Here's the drawing with two shaded views (mm, measured from the low corner). I have some questions. Coordinates: 2 decimals unless noted, no trailing zeros. Loops run counter-clockwise (first coordinate to the right, second up) from the corner with the lowest first, then second, coordinate; pieces in that order, holes last. Notation, with made-up numbers: (-0.75, 62) -> (56.25, 62) arc R19 cw to (56.25, 88) -> close; hole circle Ø11 at (-7.5, 21). An arc over 180 degrees is marked (long way). Answer as a JSON object with one key per item and string values. Group by question number.
Q1. I want a section at A-A on x = 50.8. Count the separate pieces of the cut face and the enclosed holes in it, then the cut area to 3 significant figures.
Q2. Thinking about a two-plate mould opening in Z: for the marked faces 1, 2 and 3, which applies, released by +Z, released by -Z, zero draft, split by the parting line, or undercut?
Q3. I want a section at D-D on y = 16.75. Write out the boundary of the cut face in (x, z) (3 decimals).
Q4. I need wall thicknesses on line 1 (Z direction, x = 50.8, y = 16); line 2 (Y direction, x = 50, z = 88.9) (3 decimals); line 3 (Y direction, x = 7.5, z = 50.5). Which ranges of each line are inside material? Lowest first, please.
Q5. I want a section at C-C on x = 38.5. Write out the boundary of the cut face in (y, z).
Q6. I want a section at B-B on z = 50.8. Write out the boundary of the cut face in (x, y) (3 decimals), then the cut area to 3 significant figures.
Q7. I'm going to push flat-ended pins straight in: pin 1 (4 mm diameter, centred on y = 4.5, z = 91, fed in from +X); pin 2 (10 mm diameter, centred on x = 12.7, z = 50.8, fed in from -Y); pin 3 (1.5 mm diameter, centred on y = 11, z = 47, fed in from -X); pin 4 (6.5 mm diameter, centred on y = 3.5, z = 91, fed in from -X). Where does each tip first touch, or does it pass through?
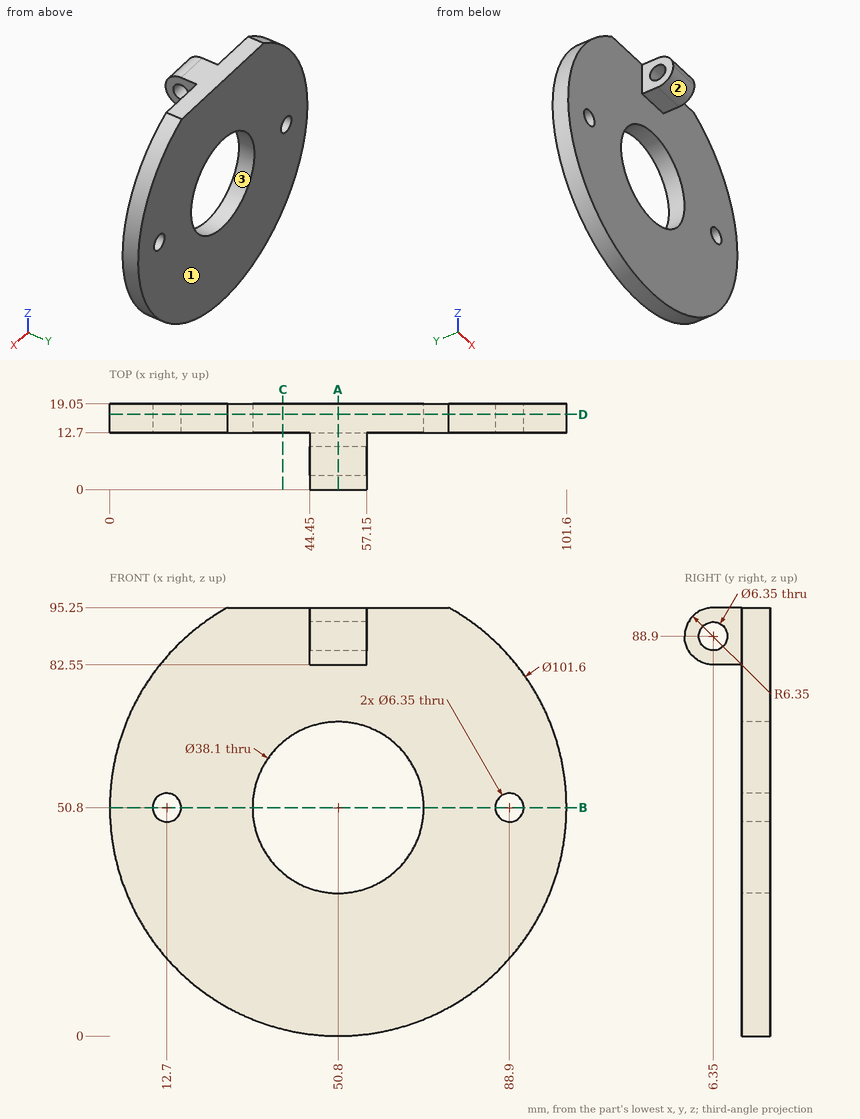
Result set:
{
 "1": {"separate pieces": "2", "enclosed holes": "1", "area": "475 mm²"},
 "2": {"face 1": "zero draft", "face 2": "released by -Z", "face 3": "undercut"},
 "3": {"outline": "(26.207, 95.25) arc R50.8 ccw (long way) to (75.393, 95.25) -> close; hole circle Ø6.35 at (12.7, 50.8); hole circle Ø38.1 at (50.8, 50.8); hole circle Ø6.35 at (88.9, 50.8)"},
 "4": {"line 1": "z = 0 to 31.75, 69.85 to 95.25", "line 2": "y = 0 to 3.175, 9.525 to 19.05", "line 3": "y = 12.7 to 19.05"},
 "5": {"outline": "(12.7, 1.51) -> (19.05, 1.51) -> (19.05, 36.25) -> (12.7, 36.25) -> close; (12.7, 65.35) -> (19.05, 65.35) -> (19.05, 95.25) -> (12.7, 95.25) -> close"},
 "6": {"outline": "(0, 12.7) -> (9.525, 12.7) -> (9.525, 19.05) -> (0, 19.05) -> close; (15.875, 12.7) -> (31.75, 12.7) -> (31.75, 19.05) -> (15.875, 19.05) -> close; (69.85, 12.7) -> (85.725, 12.7) -> (85.725, 19.05) -> (69.85, 19.05) -> close; (92.075, 12.7) -> (101.6, 12.7) -> (101.6, 19.05) -> (92.075, 19.05) -> close", "area": "323 mm²"},
 "7": {"pin 1": "stops at x = 57.15", "pin 2": "stops at y = 12.7", "pin 3": "passes through", "pin 4": "stops at x = 44.45"}
}
